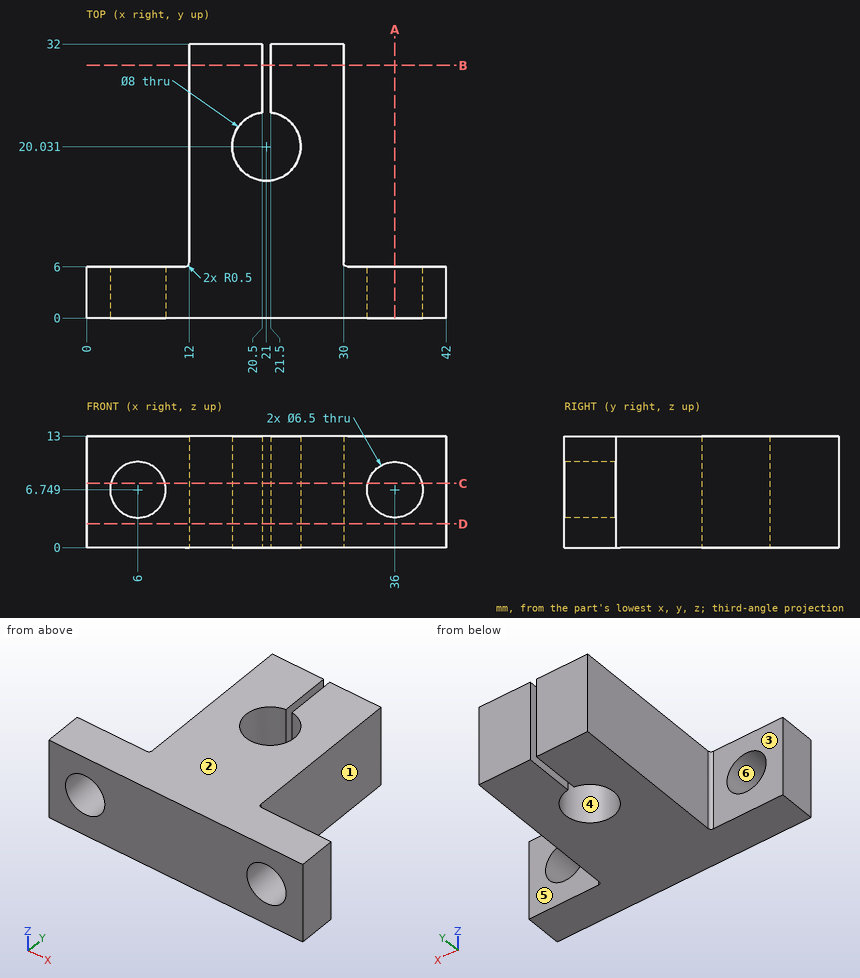
Job drawing, mm, ordinate dimensions from the low corner. One solid piece. A direction names the side the tool comes from. Give positions to 0.01 mm unless a question says otherwise; leave off trailing zeros. Order: outer loops, then holes, each group sorted by start corner. A loop starts at its lowest first (then second) coordinate and runs counter-clockwise, first axis right, second up. Notation, with made-up numbers: (-3, 53.5) - (43, 53.5) arc R20 cw to (43, 68.5) - close; hole circle Ø9 at (34.25, 27.5). An arc over 180 degrees is marked (long way). Answer in a Markdown table with one row per item.
1. Pull direction Y, two halves, no side cores. Call the marked faces 4, 5 and 6: pulls with the +Y half, pulls with the -Y half, needs draft (parallel to the pull), parting line crosses it, or undercut.
Data:
| item | result |
|---|---|
| face 4 | undercut |
| face 5 | pulls with the +Y half |
| face 6 | needs draft |
2. Saw through at B-B, the plane y = 29.5. Give the cut face in (x, z).
Data:
| item | result |
|---|---|
| outline | (12, 0) - (20.5, 0) - (20.5, 13) - (12, 13) - close; (21.5, 0) - (30, 0) - (30, 13) - (21.5, 13) - close |
3. Flat gauge pins, fed straight in: pin 1 (1.5 mm diameter, centred on x = 13.5, y = 19, fed in from -Z); pin 2 (1.5 mm diameter, centred on y = 23, z = 4, fed in from -X); pin 3 (5 mm diameter, centred on y = 10.5, z = 11, fed in from +X). Where does each tip first touch, or does it go through?
Data:
| item | result |
|---|---|
| pin 1 | stops at z = 0 |
| pin 2 | stops at x = 12 |
| pin 3 | stops at x = 30 |
4. Saw through at A-A, the plane x = 36. Give the cut face in (y, z), plus the area to 3 significant figures.
Data:
| item | result |
|---|---|
| outline | (0, 0) - (6, 0) - (6, 3.5) - (0, 3.5) - close; (0, 10) - (6, 10) - (6, 13) - (0, 13) - close |
| area | 39.0 mm² |
5. Saw through at D-D, the plane z = 2.75. Give the cut face in (x, y), plus the area to 3 significant figures.
Data:
| item | result |
|---|---|
| outline | (0, 0) - (42, 0) - (42, 6) - (30.5, 6) arc R0.5 cw to (30, 6.5) - (30, 32) - (21.5, 32) - (21.5, 24) arc R4 cw (long way) to (20.5, 24) - (20.5, 32) - (12, 32) - (12, 6.5) arc R0.5 cw to (11.5, 6) - (0, 6) - close |
| area | 662 mm² |
6. Probe probe 1 along X at (y, z) = (3.5, 6.5); probe 2 along X at (y, z) = (26, 11.25); probe 3 along Z at (x, y) = (6, 1.5). List the from-to ranges inside material, lowest first. Write a range as [from, to].
Data:
| item | result |
|---|---|
| probe 1 | x = [0, 2.76], [9.24, 32.76], [39.24, 42] |
| probe 2 | x = [12, 20.5], [21.5, 30] |
| probe 3 | z = [0, 3.5], [10, 13] |
7. Tool access for the marked faces 1, 2 and 3: list every direction of +Z, -Z, +X, -X, +Y, -Y with a clear straight run to the whole face (end or side of a thin tool).
Data:
| item | result |
|---|---|
| face 1 | +Z, -Z, +X, +Y |
| face 2 | +Z, +X, -X, +Y, -Y |
| face 3 | +Z, -Z, -X, +Y |
8. Saw through at C-C, the plane z = 7.5. Give the cut face in (x, y).
Data:
| item | result |
|---|---|
| outline | (0, 0) - (2.84, 0) - (2.84, 6) - (0, 6) - close; (9.16, 0) - (32.84, 0) - (32.84, 6) - (30.5, 6) arc R0.5 cw to (30, 6.5) - (30, 32) - (21.5, 32) - (21.5, 24) arc R4 cw (long way) to (20.5, 24) - (20.5, 32) - (12, 32) - (12, 6.5) arc R0.5 cw to (11.5, 6) - (9.16, 6) - close; (39.16, 0) - (42, 0) - (42, 6) - (39.16, 6) - close |
